Autodesk Inventor part; units mm, degrees
ref_plane "YZ Plane" through (0, 0, 0) normal (1, 0, 0) x (0, 1, 0)
ref_plane "XZ Plane" through (0, 0, 0) normal (0, 1, 0) x (-1, 0, 0)
ref_plane "XY Plane" through (0, 0, 0) normal (0, 0, 1) x (1, 0, 0)
sketch "Sketch1" plane through (0, 0, 0) normal (0, 0, 1) x (1, 0, 0)
  arc A0 (-1.9795, 6.7143) -> (1.9795, 6.7143) centre (0, 7) ccw
  arc A1 (-1.9795, 6.7143) -> (-1.9795, -6.7143) centre (0, 0) ccw
  arc A2 (1.9795, -6.7143) -> (-1.9795, -6.7143) centre (0, -7) ccw
  arc A3 (1.9795, -6.7143) -> (1.9795, 6.7143) centre (0, 0) ccw
  line L0 (3.6, 1.9621) -> (3.6, -1.9621)
  arc A4 (3.6, 1.9621) -> (3.6, -1.9621) centre (0, 0) ccw
  circle A5 centre (0, -7) radius 1.75
  circle A6 centre (0, 7) radius 1.75
  circle A7 centre (0, 0) radius 7.5
  circle A8 centre (0, 0) radius 102.5
  point P0 (0, 0)
  point P1 (-1.7242, 7.2991)
  point P2 (1.7242, 7.2991)
  point P3 (1.7242, -7.2991)
  point P4 (-1.7242, -7.2991)
  dimension "d0" = 3.5
  dimension "d1" = 3.5
  dimension "d2" = 15
  dimension "d3" = 205
extrude "Extrusion1" add sketch "Sketch1" against normal blind 8.25 contours A5 A7 | A7 A5 | A7 A6 | A6 A7 | A8
fillet "Fillet1" radius 3.5 1 edges at (-102.5, 0, -8.25)
sketch "Sketch2" plane through (0, 0, 0) normal (0, 0, 1) x (1, 0, 0)
  circle A0 centre (0, 0) radius 5.25
  arc A1 (1.7242, -7.2991) -> (-1.7242, -7.2991) centre (0, -7) ccw
  circle A2 centre (0, 0) radius 10
  circle A3 centre (0, 0) radius 102.5
  dimension "d7" = 20
extrude "Extrusion2" add sketch "Sketch2" along normal blind 4 contours A2 | A3
sketch "Sketch3" plane through (0, 0, 4) normal (0, 0, 1) x (1, 0, 0)
  circle A0 centre (0, 0) radius 5.25
  arc A1 (1.7242, -7.2991) -> (1.7242, 7.2991) centre (0, 0) ccw
  circle A2 centre (0, 0) radius 1.4142
  circle A3 centre (0, 0) radius 3.6056
  arc A4 (0, -5.25) -> (0, 5.25) centre (0, 0) ccw
  arc A5 (1.7242, -7.2991) -> (1.7242, 7.2991) centre (0, 0) ccw
  circle A6 centre (0, 0) radius 7.5
  point P0 (1.7242, 7.2991)
extrude "Extrusion3" add sketch "Sketch3" along normal blind 4 contours A0 | A6 A1 | A3
sketch "Sketch4" plane through (0, 0, 8) normal (0, 0, 1) x (1, 0, 0)
  circle A0 centre (0, 0) radius 4
extrude "Extrusion4" cut sketch "Sketch4" against normal blind 2
sketch "Sketch5" plane through (0, 0, 0) normal (1, 0, 0) x (0, 1, 0)
  line L0 (102.5, 4) -> (-102.5, 4)
  line L1 (-102.5, -4.75) -> (102.5, -4.75)
  line L2 (7.5, 8) -> (-7.5, 8)
  line L3 (-7.5, 4) -> (7.5, 4)
  line L4 (7.5, 4) -> (17.5, 4)
  line L5 (17.5, 4) -> (102.5, -4.75)
  line L6 (102.5, -4.75) -> (102.5, 16)
  line L7 (102.5, 16) -> (7.5, 16)
  line L8 (7.5, 16) -> (7.5, 4)
  line L9 (0, -13.1) -> (0, 20.85)
  point P0 (0, 0)
  dimension "d14" = 10
revolve "Revolution1" cut sketch "Sketch5" angle 360 about axis through (0, 0, -10) along (0, 0, 1) contours L6 L5 L0 | L0 L8 L7 L6
properties part number "center_disk"
Verification items for the finished model (mm, model axes). A direction names the side the tool comes from. Give positions to 0.01 mm unless a question says otherwise; leave off trailing zeros. Use a Markdown table: item, result.
1) Material ranges on probe 1 along Y at (x, z) = (0, 5.5); probe 2 along Y at (x, z) = (0, 7.2); probe 3 along Z at (x, y) = (-55, 49), recorded low to high.
Results:
| item | result |
|---|---|
| probe 1 | -7.5 to -1.41, 1.41 to 7.5 |
| probe 2 | -7.5 to -4, 4 to 7.5 |
| probe 3 | -8.25 to -1.78 |
2) Mould release check, pull along X, two halves, no side actions. Record for faces 1 (the flat face through (0, -8, 4)), 2 (the cylindrical face through (7.5, -0.1, -4.1)), 3 (the cylindrical face through (-7.498, -0.189, 5.972)): pulls with the +X half, pulls with the -X half, needs draft (parallel to the pull), parting line crosses it, or undercut.
Results:
| item | result |
|---|---|
| face 1 | needs draft |
| face 2 | undercut |
| face 3 | parting line crosses it |
3) Depth check by flat-ended pin: pin 1 Ø6.5 at (x, y) = (0, 0) entering from +Z; pin 2 Ø6 at (y, z) = (-18, -6) entering from +X; pin 3 Ø8 at (y, z) = (39.5, -4.5) entering from -X; pin 4 Ø8.5 at (x, y) = (1.5, -2) entering from -Z. Enter the tip coordinate at first touch or a pass-through.
Results:
| item | result |
|---|---|
| pin 1 | z = 6 |
| pin 2 | x = 101.36 |
| pin 3 | x = -96.15 |
| pin 4 | z = -8.25 |
4) Tool access check on faces 4 (the flat face through (2, 0, 6)), 5 (the cylindrical face through (7.5, 0.1, 6)), 6 (the flat face through (3, -3, 8)), 7 (the cylindrical face through (5, -1.6, 2)). Record the directions out of +Z, -Z, +X, -X, +Y, -Y that give a thin tool (end or side, any length) a straight path to the whole face; none if there is none.
Results:
| item | result |
|---|---|
| face 4 | +Z |
| face 5 | +Z, +X |
| face 6 | +Z, +X, -X, +Y, -Y |
| face 7 | -Z |
